CAD build for the part. Positions are in the model's coordinates, mm. A direction names the side the tool comes from. Round coordinates to 2 decimals unless told otherwise and drop trailing zeros. Order: outer loops, then holes, each group sorted by start corner. A loop starts at its lowest first (then second) coordinate and runs counter-clockwise, first axis right, second up. Notation, with made-up numbers: (45.25, 26) -> (70.25, 26) arc R22 ccw to (70.25, 39) -> close; hole circle Ø4 at (27.5, 5.25). An arc over 180 degrees is marked (long way). Return JSON: item names as keys, results as strings. Group by question number.
Q1. Cut at A-A (y = 15). Write the cut outline in (x, z), then the cut area to 3 significant figures.
Q2. Cut at C-C (x = -32). Write the cut outline in (y, z).
Q3. Cut at B-B (x = -56). Write the cut outline in (y, z), then the cut area to 3 significant figures.
Q4. Cut at D-D (z = -2.5). Write the cut outline in (x, y), then the cut area to 3 significant figures.
Q5. Mould opens along X. For faces 1 (the cylindrical face through (-50, 5, -5)), 2 (the flat face through (-56, 0, -1)), 3 (the cylindrical face through (-60.37, 10.14, -4.36)), 4 (the flat face through (-29.65, 13, -10)) say: +X half, -X half, draft (parallel to the pull), parting line (faces both ways), or undercut.
Q6. Probe line 1 along Y through (x, z) = (-56, -0.25); line 2 along Z through (x, y) = (-33, 7.75); line 3 along Y through (x, z) = (-28, -2.5). List the from-to ranges inside material, lowest first.
Q7. Which spindle directions (+Z, -Z, +X, -X, +Y, -Y) get a long thin tool onto all of the face, cutting with end or side? Do faces 5 (the flat face through (-25.65, 13, -6)), 6 (the flat face through (-51, 1, -3)), 7 (the flat face through (-33, 13, -6.15)). Say none if no direction does.
Q8. Flat gauge pins, fed straight in: pin 1 (8 mm diameter, centred on x = -45, y = 16.5, fed in from -Z); pin 2 (8.5 mm diameter, centred on y = 15.5, z = -12, fed in from -X); pin 3 (4 mm diameter, centred on x = -56, y = 13, fed in from -Z). Where does each tip first touch, or does it go through?
from build123d import *

# Parameters (mm, degrees)
ESQUISSE2_W             = 5.7
ESQUISSE2_H             = 7.7
BOSS_EXTRU_1_DEPTH      = 20
ESQUISSE3_R             = 1.25
ESQUISSE3_R_2           = 1
ESQUISSE3_W             = 25.35
ESQUISSE3_H             = 7
ENL_V_MAT_EXTRU_1_DEPTH = 23.85
CONG_1_R                = 5
CONG_2_R                = 5


with BuildPart() as part:
    # Esquisse2 → Boss.-Extru.1 (new body)
    with BuildSketch(Plane(origin=(0, 0, 0), x_dir=(1, 0, 0), z_dir=(0, 1, 0))):
        Polygon((-61, -5), (-51.584269114, -5), (-25.65, -5), (-25.65, 17.85), (-39.35, 17.85), (-61, 4.750279551), align=None)
        with Locations((-32.5, 10)):
            Rectangle(ESQUISSE2_W, ESQUISSE2_H, mode=Mode.SUBTRACT)
    extrude(amount=BOSS_EXTRU_1_DEPTH)

    # Esquisse3 → Enlèv. mat.-Extru.1 (cut, through all)
    with BuildSketch(Plane.XY.offset(5)):
        with Locations((-56, 12.999901199)):
            Circle(ESQUISSE3_R)
        with Locations((-56, 5.999901199)):
            Circle(ESQUISSE3_R_2)
        with Locations((-38.325, 3.5)):
            Rectangle(ESQUISSE3_W, ESQUISSE3_H)
    extrude(amount=-ENL_V_MAT_EXTRU_1_DEPTH, mode=Mode.SUBTRACT)

    # Congé1
    cong_1_edges = [part.edges().sort_by_distance(p)[0] for p in [
        (-51, 7, -2.900479371),
    ]]
    fillet(cong_1_edges, radius=CONG_1_R)

    # Congé2
    cong_2_edges = [part.edges().sort_by_distance(p)[0] for p in [
        (-61, 10, -4.750279551),
        (-39.35, 13.5, -17.85),
    ]]
    fillet(cong_2_edges, radius=CONG_2_R)


solid = part.part
Solution:
{
 "1": {"outline": "(-61, -1.93) arc R5 ccw to (-58.59, -6.21) -> (-40.54, -17.13) arc R5 ccw to (-37.96, -17.85) -> (-25.65, -17.85) -> (-25.65, 5) -> (-61, 5) -> close; hole (-35.35, -13.85) -> (-29.65, -13.85) -> (-29.65, -6.15) -> (-35.35, -6.15) -> close", "area": "621 mm²"},
 "2": {"outline": "(7, -17.85) -> (20, -17.85) -> (20, -13.85) -> (7, -13.85) -> close; (7, -6.15) -> (20, -6.15) -> (20, 5) -> (7, 5) -> close"},
 "3": {"outline": "(0, -7.78) -> (5, -7.78) -> (5, 5) -> (0, 5) -> close; (7, -7.78) -> (11.75, -7.78) -> (11.75, 5) -> (7, 5) -> close; (14.25, -7.78) -> (20, -7.78) -> (20, 5) -> (14.25, 5) -> close", "area": "198 mm²"},
 "4": {"outline": "(-60.97, 0) -> (-51, 0) -> (-51, 2) arc R5 cw to (-46, 7) -> (-25.65, 7) -> (-25.65, 20) -> (-60.97, 20) -> close; hole circle Ø2.5 at (-56, 13); hole circle Ø2 at (-56, 6)", "area": "526 mm²"},
 "5": {"face 1": "+X half", "face 2": "draft", "face 3": "-X half", "face 4": "undercut"},
 "6": {"line 1": "y = 0 to 5, 7 to 11.75, 14.25 to 20", "line 2": "z = -17.85 to -13.85, -6.15 to 5", "line 3": "y = 7 to 20"},
 "7": {"face 5": "+Z, -Z, +X, +Y, -Y", "face 6": "+Z, -Z, +X, -Y", "face 7": "+Y, -Y"},
 "8": {"pin 1": "stops at z = -16.85", "pin 2": "stops at x = -56.04", "pin 3": "stops at z = -8.99"}
}
